from build123d import *

# Parameters (mm, degrees)
BOSS_EXTRUDE1_DEPTH = 3.175
SKETCH2_W           = 222.25
SKETCH2_H           = 3.175
CUT_EXTRUDE1_DEPTH  = 4.175
SKETCH3_W           = 25.4
SKETCH3_H           = 25.4
CUT_EXTRUDE2_DEPTH  = 10


with BuildPart() as part:
    # Sketch1 → Boss-Extrude1 (new body)
    with BuildSketch(Plane(origin=(0, 0, 0), x_dir=(0, 0, -1), z_dir=(1, 0, 0))):
        Polygon((-116.659983875, 27.078998721), (-116.659983875, 1.678998721), (-119.834983875, 1.678998721), (-119.834983875, -23.721001279), (-116.659983875, -23.721001279), (-116.659983875, -42.771001279), (-65.859983875, -42.771001279), (-65.859983875, -45.946001279), (-40.459983875, -45.946001279), (-40.459983875, -42.771001279), (29.390016125, -42.771001279), (29.390016125, -45.946001279), (54.790016125, -45.946001279), (54.790016125, -42.771001279), (105.590016125, -42.771001279), (105.590016125, -23.721001279), (108.765016125, -23.721001279), (108.765016125, 1.678998721), (105.590016125, 1.678998721), (105.590016125, 27.078998721), align=None)
    extrude(amount=BOSS_EXTRUDE1_DEPTH)

    # Sketch2 → Cut-Extrude1 (cut, through all)
    with BuildSketch(Plane(origin=(3.175, 0, 0), x_dir=(0, 0, -1), z_dir=(1, 0, 0))):
        with Locations((-5.534983875, 25.491498721)):
            Rectangle(SKETCH2_W, SKETCH2_H)
    extrude(amount=-CUT_EXTRUDE1_DEPTH, mode=Mode.SUBTRACT)

    # Sketch3 → Cut-Extrude2 (cut)
    with BuildSketch(Plane.ZY):
        with Locations((58.843980592, -5.975859027)):
            Rectangle(SKETCH3_W, SKETCH3_H)
    extrude(amount=-CUT_EXTRUDE2_DEPTH, mode=Mode.SUBTRACT)


solid = part.part
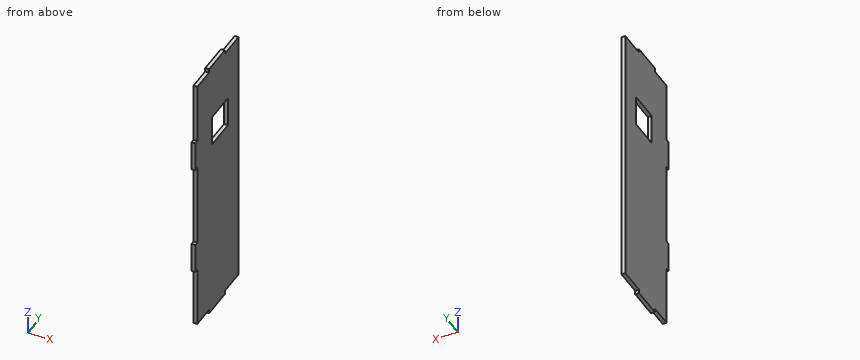
The model under review builds one solid part; all positions refer to its coordinate system, in mm. Give positions to 0.01 mm unless a question says otherwise; leave off trailing zeros. Order: outer loops, then holes, each group sorted by start corner. A loop starts at its lowest first (then second) coordinate and runs counter-clockwise, first axis right, second up. Notation, with made-up numbers: M -31,51.5 L 2,51.5 A17 ccw 2,55.5 Z; hole C 33.5,36.5 d11. An arc over 180 degrees is marked long. Answer in a Markdown table with one row per item. Add a question column.
1. Add section B-B on z = 56. State the section outline as (x, y) points (3 decimals), plus the area to 3 significant figures.
2. To check wall thickness, follow line 1 along Y through (x, z) = (0.3, 66.5); line 2 along Y through (x, z) = (2.7, 29.5); line 3 along Z through (x, y) = (1.95, 5.5). State the ranges of each line that lie inside material, in increasing order.
3. Add section D-D on z = 25.5. State the section outline as (x, y) points (3 decimals).
4. Add section C-C on x = 2.15. State the section outline as (y, z) points.
5. For pin 1 Ø1.6 at (x, y) = (2.5, -33.5) entering from +Z; pin 2 Ø1 at (x, y) = (2, -30) entering from -Z; pin 3 Ø1.6 at (x, z) = (2, -107) entering from +Y, all flat-tipped, find the tip position at first contact; note any pin that passes through.
6. Add section A-A on y = 4. State the section outline as (x, z) points (3 decimals).
The answers:
| question | item | result |
|---|---|---|
| 1 | outline | M 0,-45.946 L 3.175,-45.946 L 3.175,-18.676 L 0,-18.676 Z; M 0,6.724 L 3.175,6.724 L 3.175,23.904 L 0,23.904 Z |
| 1 | area | 141 mm2 |
| 2 | line 1 | -42.77 to -18.68, 6.72 to 23.9 |
| 2 | line 2 | -42.77 to 23.9 |
| 2 | line 3 | -105.59 to 46.14, 71.54 to 116.66 |
| 3 | outline | M 0,-42.771 L 3.175,-42.771 L 3.175,23.904 L 0,23.904 Z |
| 4 | outline | M -45.95,-54.79 L -42.77,-54.79 L -42.77,-105.59 L -23.72,-105.59 L -23.72,-108.77 L 1.68,-108.77 L 1.68,-105.59 L 23.9,-105.59 L 23.9,116.66 L 1.68,116.66 L 1.68,119.83 L -23.72,119.83 L -23.72,116.66 L -42.77,116.66 L -42.77,65.86 L -45.95,65.86 L -45.95,40.46 L -42.77,40.46 L -42.77,-29.39 L -45.95,-29.39 Z; hole M -18.68,46.14 L 6.72,46.14 L 6.72,71.54 L -18.68,71.54 Z |
| 5 | pin 1 | z = 116.66 |
| 5 | pin 2 | z = -105.59 |
| 5 | pin 3 | y = 1.68 |
| 6 | outline | M 0,-105.59 L 3.175,-105.59 L 3.175,46.144 L 0,46.144 Z; M 0,71.544 L 3.175,71.544 L 3.175,116.66 L 0,116.66 Z |
